Autodesk Inventor part; units mm, degrees
ref_plane "YZ Plane" through (0, 0, 0) normal (1, 0, 0) x (0, 1, 0)
ref_plane "XZ Plane" through (0, 0, 0) normal (0, 1, 0) x (-1, 0, 0)
ref_plane "XY Plane" through (0, 0, 0) normal (0, 0, 1) x (1, 0, 0)
sketch "Sketch2" plane through (0, 0, 0) normal (0, 0, 1) x (1, 0, 0)
  line L0 (0, 0) -> (133.35, 0)
  line L1 (133.35, 0) -> (133.35, 57.15)
  line L2 (0, 57.15) -> (0, 0)
  line L3 (0, 57.15) -> (6.35, 57.15)
  line L4 (6.35, 57.15) -> (6.35, 50.8)
  line L5 (6.35, 50.8) -> (12.7, 50.8)
  line L6 (12.7, 50.8) -> (12.7, 57.15)
  line L7 (12.7, 57.15) -> (19.05, 57.15)
  line L8 (19.05, 57.15) -> (19.05, 50.8)
  line L9 (19.05, 50.8) -> (25.4, 50.8)
  line L10 (25.4, 50.8) -> (25.4, 57.15)
  line L11 (25.4, 57.15) -> (31.75, 57.15)
  line L12 (31.75, 57.15) -> (31.75, 50.8)
  line L13 (31.75, 50.8) -> (38.1, 50.8)
  line L14 (38.1, 50.8) -> (38.1, 57.15)
  line L15 (38.1, 57.15) -> (44.45, 57.15)
  line L16 (44.45, 57.15) -> (44.45, 50.8)
  line L17 (44.45, 50.8) -> (50.8, 50.8)
  line L18 (50.8, 50.8) -> (50.8, 57.15)
  line L19 (50.8, 57.15) -> (57.15, 57.15)
  line L20 (57.15, 57.15) -> (57.15, 50.8)
  line L21 (57.15, 50.8) -> (63.5, 50.8)
  line L22 (63.5, 50.8) -> (63.5, 57.15)
  line L23 (63.5, 57.15) -> (69.85, 57.15)
  line L24 (69.85, 57.15) -> (69.85, 50.8)
  line L25 (69.85, 50.8) -> (76.2, 50.8)
  line L26 (76.2, 50.8) -> (76.2, 57.15)
  line L27 (76.2, 57.15) -> (82.55, 57.15)
  line L28 (82.55, 57.15) -> (82.55, 50.8)
  line L29 (82.55, 50.8) -> (88.9, 50.8)
  line L30 (88.9, 50.8) -> (88.9, 57.15)
  line L31 (88.9, 57.15) -> (95.25, 57.15)
  line L32 (95.25, 57.15) -> (95.25, 50.8)
  line L33 (95.25, 50.8) -> (101.6, 50.8)
  line L34 (101.6, 50.8) -> (101.6, 57.15)
  line L35 (101.6, 57.15) -> (107.95, 57.15)
  line L36 (107.95, 57.15) -> (107.95, 50.8)
  line L37 (107.95, 50.8) -> (114.3, 50.8)
  line L38 (114.3, 50.8) -> (114.3, 57.15)
  line L39 (114.3, 57.15) -> (120.65, 57.15)
  line L40 (120.65, 57.15) -> (120.65, 50.8)
  line L41 (120.65, 50.8) -> (127, 50.8)
  line L42 (127, 50.8) -> (127, 57.15)
  line L43 (127, 57.15) -> (133.35, 57.15)
  dimension "Length" = 133.35
  dimension "Height" = 57.15
  dimension "Teeth_Width" = 6.35
  dimension "Material_Thickness" = 6.35
  dimension "d63" = 6.35
  dimension "d64" = 6.35
  dimension "d65" = 6.35
  dimension "d66" = 6.35
  dimension "d67" = 6.35
  dimension "d68" = 6.35
  dimension "d69" = 6.35
  dimension "d70" = 6.35
  dimension "d71" = 6.35
  dimension "d72" = 6.35
  dimension "d73" = 6.35
  dimension "d74" = 6.35
  dimension "d75" = 6.35
  dimension "d76" = 6.35
  dimension "d77" = 6.35
  dimension "d78" = 6.35
  dimension "d79" = 6.35
  dimension "d80" = 6.35
  dimension "d81" = 6.35
  dimension "d82" = 6.35
  dimension "d83" = 6.35
  dimension "d84" = 6.35
  dimension "d85" = 6.35
  dimension "d86" = 6.35
  dimension "d87" = 6.35
  dimension "d88" = 6.35
  dimension "d89" = 6.35
  dimension "d90" = 6.35
extrude "Extrusion2" add sketch "Sketch2" along normal blind 6.35
equation "\"d63\" = Teeth_Width"
equation "\"d66\" = d64"
equation "\"d69\" = d67"
equation "\"d72\" = d70"
equation "\"d75\" = d73"
equation "\"d78\" = d76"
equation "\"d81\" = d79"
equation "\"d84\" = d82"
equation "\"d87\" = d85"
equation "\"d90\" = d88"
properties part number "Side Support"
The model under review builds one solid part; all positions refer to its coordinate system, in mm. A direction names the side the tool comes from. Round coordinates to 2 decimals unless told otherwise and drop trailing zeros. Order: outer loops, then holes, each group sorted by start corner. A loop starts at its lowest first (then second) coordinate and runs counter-clockwise, first axis right, second up. Notation, with made-up numbers: (69, 87) -> (99, 87) arc R16 ccw to (99, 118) -> close; hole circle Ø10 at (-16, -36.5). An arc over 180 degrees is marked (long way). One line per item, written item: value. Start each with the question number.
Q1. Wall thickness on line 1 (Y direction, x = 50.5, z = 3): over which ranges is the line inside the solid? List them lowest first.
Q2. Machinability: for faces 4 (the face through (16, 57.15, 3)), 5 (the face through (60, 50.8, 3)), which of the approach directions +Z, -Z, +X, -X, +Y, -Y give a long, thin tool a straight path to every point of the face, cutting with its end or side? Answer none if there is none.
Q3. Clearance check with flat-ended pins moving along their axes: pin 1 Ø3 at (x, z) = (58, 3.5) entering from -Y; pin 2 Ø1.9 at (x, z) = (124, 4.5) entering from +Y. State where each tip first meets the part, or that it passes through.
Q4. Take a section at A-A (x = 35.5). Write out the cut boundary in (y, z), and give its area (3 significant figures).
Q5. Mouldability with a two-part tool opening along X and no side actions: class faces 1 (the face through (0, 29, 3)), 2 (the face through (66, 0, 3)), 3 (the face through (76.2, 54, 3)) as released by +X, released by -X, zero draft, split by the parting line, or undercut.
Reported:
1. line 1: y = 0 to 50.8
2. face 4: +Z, -Z, +X, -X, +Y
2. face 5: +Z, -Z, +Y
3. pin 1: stops at y = 0
3. pin 2: stops at y = 50.8
4. outline: (0, 0) -> (50.8, 0) -> (50.8, 6.35) -> (0, 6.35) -> close
4. area: 323 mm2
5. face 1: released by -X
5. face 2: zero draft
5. face 3: undercut
